Autodesk Fusion 360 part; units mm, degrees
sketch "Sketch1" plane through (0, 0, 0) normal (1, 0, 0) x (0, 1, 0) in component "Wheel v0"
  line L0 (0, 0) -> (9.2, 0)
  line L1 (9.2, 0) -> (9.2, 12)
  line L2 (9.2, 12) -> (0, 12)
  line L3 (0, 12) -> (0, 0)
  line L4 (0, 10.3) -> (9.2, 10.3)
  line L5 (7.1, 0) -> (8.3, 0)
  line L6 (8.3, 0) -> (8.3, 1.2)
  line L7 (8.3, 1.2) -> (7.1, 1.2)
  line L8 (7.1, 1.2) -> (7.1, 0)
  circle A0 centre (3.6, 0) radius 2.6
  line L9 (3.6, 0) -> (3.6, 2.6) construction
  circle A1 centre (3.6, 2.6) radius 0.5
  dimension "d1" = 9.2
  dimension "d2" = 12
  dimension "d3" = 1.7
  dimension "d4" = 1.2
  dimension "d5" = 1.2
  dimension "d6" = 7.1
  dimension "d7" = 5.2
  dimension "d8" = 3.6
  dimension "d9" = 1
revolve "Revolve1" add sketch "Sketch1" angle 360 about axis through (0, 9.2, 12) along (0, -1, 0) contours L0 L1 L3 L4 L6 L7 L8 A0 A1 | L1 L2 L3 L4 in component "Wheel v0"
chamfer "Chamfer1" distance 0.6 angle 45 2 faces at (-0.5962, 7.1, 0.4447) (-1.1327, 8.3, 0.4849) in component "Wheel v0"
chamfer "Chamfer1" distance 0.1 angle 45 2 edges at (-11.1879, 9.2, 7.6606) (-11.1879, 0, 7.6606) in component "Wheel v0"
chamfer "Chamfer1" distance 0.28 distance2 0.31 2 edges at (-8.8087, 4.0977, 8.5834) (-8.8087, 3.1023, 8.5834) measured on face at (-0.4697, 4.0994, 21.4123) measured on face at (7.1736, 1.0027, 21.4704) in component "Wheel v0"
chamfer "Chamfer1" distance 0.32 distance2 0.3 2 edges at (-11.1879, 6.2, 7.6606) (-11.1879, 1, 7.6606) measured on face at (-1.1829, 6.1973, 23.8216) measured on face at (-0.5982, 0.3333, 0.0149) in component "Wheel v0"
sketch "Sketch2" plane through (0, 0, 0) normal (0, -1, 0) x (1, 0, 0) in component "Wheel v0"
  circle A0 centre (0, 12) radius 11.9
  circle A1 centre (0, 12) radius 1.6
  line L0 (-1.2072, 13.0501) -> (1.2072, 13.0501)
  line L1 (0.0188, 10.4001) -> (0, 0) construction
  circle A2 centre (0, 12) radius 1.4
  dimension "d17" = 3.2
  dimension "d18" = 2.65
  dimension "d19" = 2.8
extrude "Extrude6" cut sketch "Sketch2" against normal blind 9.2 contours A1 L0 A2 | L0 A2 picked at (-1.0596, 13.1037) picked at (-0.2497, 13.1644) in component "Wheel v0"
component "Wheel v0" placed x (0, 1, 0) y (1, 0, 0) z (0, 0, -1) at (44.7, 15, 25.75)
Check sheet for the modelled part. Datum: model origin and axes. Units: mm. Coordinates: 2 decimals unless noted, no trailing zeros. Answer as CSV lines item,"result".
Q1. Go/stop test with flat-tipped pins: pin 1 (5 mm diameter, centred on x = 46.5, z = 18, fed in from -Y); pin 2 (0.7 mm diameter, centred on x = 49.5, y = 15, fed in from -Z). Record where each tip stops, or that it passes through.
Check result:
pin 1,"y = 3.17"
pin 2,"z = 3.84"
Q2. Material ranges on probe 1 along X at (y, z) = (4.25, 15.5); probe 2 along Z at (x, y) = (51, 13.5); probe 3 along X at (y, z) = (21, 4.5), recorded low to high. Write a range as from..to.
Check result:
probe 1,"44.7..45.95, 50.65..52.31, 52.49..53.9"
probe 2,"2.05..25.45"
probe 3,"44.7..45.89, 50.71..52.17, 52.63..53.9"
Q3. Mould release check, pull along Y, two halves, no side actions. Record for faces 1 (the face through (49.24, 15.02, 12.15)), 2 (the face through (53.9, 15, 14)), 3 (the face through (45.094, 6.89, 4.906)), 4 (the face through (49, 15, 12.7)): released by +Y, released by -Y, zero draft, split by the parting line, or undercut.
Check result:
face 1,"undercut"
face 2,"zero draft"
face 3,"split by the parting line"
face 4,"undercut"
